from build123d import *

# Parameters (mm, degrees)
PAD_DEPTH         = 50
SKETCH001_W       = 0.9
SKETCH001_H       = 10
POCKET_DEPTH      = 10.001
POCKET_DEPTH_BACK = -10.001
CHAMFER_SIZE      = 1
CHAMFER001_SIZE   = 0.5


with BuildPart() as part:
    # Sketch → Pad (new body)
    with BuildSketch(Plane.YZ):
        with BuildLine():
            Line((-10, 0), (10, 0))
            Line((10, 0), (7.5, 10))
            Line((7.5, 10), (2.3, 10))
            Line((2.3, 10), (1.906144, 6.463458))
            ThreePointArc((1.906144, 6.463458), (1.913219, 6.190714), (1.99375, 5.930033))
            ThreePointArc((-1.99375, 5.930033), (0, 2.8), (1.99375, 5.930033))
            ThreePointArc((-1.99375, 5.930033), (-1.913219, 6.190714), (-1.906144, 6.463458))
            Line((-1.906144, 6.463458), (-2.3, 10))
            Line((-2.3, 10), (-7.5, 10))
            Line((-7.5, 10), (-10, 0))
        make_face()
    extrude(amount=PAD_DEPTH)

    # Sketch001 → Pocket (cut, two sides)
    with BuildSketch(Plane.XZ) as pocket_sk:
        with Locations((10.45, 7)):
            Rectangle(SKETCH001_W, SKETCH001_H)
    extrude(amount=-POCKET_DEPTH, mode=Mode.SUBTRACT)
    extrude(pocket_sk.sketch, amount=-POCKET_DEPTH_BACK, mode=Mode.SUBTRACT)

    # Chamfer
    chamfer_edges = [part.edges().sort_by_distance(p)[0] for p in [
        (25, 10, 0),
        (25, -10, 0),
    ]]
    chamfer(chamfer_edges, length=CHAMFER_SIZE)

    # Chamfer001
    chamfer001_edges = [part.edges().sort_by_distance(p)[0] for p in [
        (50, -8.628732, 5.485071),
        (50, -9.378732, 0.485071),
        (50, -4.9, 10),
        (50, 0, 0),
        (50, -2.103072, 8.231729),
        (50, 9.378732, 0.485071),
        (50, -1.913219, 6.190714),
        (50, 8.628732, 5.485071),
        (50, 0, 2.8),
        (50, 4.9, 10),
        (50, 1.913219, 6.190714),
        (50, 2.103072, 8.231729),
        (0, -8.628732, 5.485071),
        (0, -9.378732, 0.485071),
        (0, -4.9, 10),
        (0, 0, 0),
        (0, -2.103072, 8.231729),
        (0, 9.378732, 0.485071),
        (0, -1.913219, 6.190714),
        (0, 8.628732, 5.485071),
        (0, 0, 2.8),
        (0, 4.9, 10),
        (0, 1.913219, 6.190714),
        (0, 2.103072, 8.231729),
        (5, -7.5, 10),
        (10, -4.9, 10),
        (5, -2.3, 10),
        (5, 2.3, 10),
        (10, 4.9, 10),
        (5, 7.5, 10),
        (10.9, 4.9, 10),
        (30.45, 2.3, 10),
        (30.45, 7.5, 10),
        (10.9, -4.9, 10),
        (30.45, -7.5, 10),
        (30.45, -2.3, 10),
        (10, -8.5, 6),
        (10, 8.5, 6),
        (10.9, 8.5, 6),
        (10.9, -8.5, 6),
    ]]
    chamfer(chamfer001_edges, length=CHAMFER001_SIZE)


solid = part.part
Model file for the job. Use its own axes, mm. A direction names the side the tool comes from. Give positions to 0.01 mm unless a question says otherwise; leave off trailing zeros. Loops run counter-clockwise (first coordinate to the right, second up) from the corner with the lowest first, then second, coordinate; pieces in that order, holes last.
1) Pull direction X, two halves, no side cores. Call faces 4 (the flat face through (30, -5, 10)), 5 (the flat face through (11.146, 8.315, 5.696)), 6 (the flat face through (49.754, 9.174, 0.634)): +X half, -X half, draft (parallel to the pull), parting line (faces both ways), or undercut.
2) Wall check: line 1 (X direction, y = 4.25, z = 8.25); line 2 (Y direction, x = 8, z = 5); line 3 (Z direction, x = 38, y = 0). Give the ranges that are in metal, low to high.
3) Saw through at C-C (y = -3.25). Write the cut outline in (x, z), plus the area to 3 significant figures.
4) Saw through at A-A (z = 5). Write the cut outline in (x, y), plus the area to 3 significant figures.
5) Tool access for faces 1 (the flat face through (0, 0, 2)), 2 (the flat face through (5.184, -2.073, 7.962)), 3 (the flat face through (10, 2.1, 6.5)): list every direction of +Z, -Z, +X, -X, +Y, -Y with a clear straight run to the whole face (end or side of a thin tool).
6) Saw through at B-B (x = 13.5). Write the cut outline in (y, z).
7) Saw through at D-D (z = 8.25). Write the cut outline in (x, y).
8) Flat gauge pins, fed straight in: pin 1 Ø6 at (x, z) = (40, 8.5) entering from +Y (3 decimals); pin 2 Ø1 at (x, z) = (6.5, 8.5) entering from +Y; pin 3 Ø4 at (x, y) = (34, -1.5) entering from +Z; pin 4 Ø2 at (x, z) = (16, 7) entering from +Y. Where does each tip first touch, or does it go through?
Answer block:
1. face 4: draft
1. face 5: undercut
1. face 6: +X half
2. line 1: x = 0 to 10, 10.9 to 50
2. line 2: y = -8.75 to -2.2, 2.2 to 8.75
2. line 3: z = 0 to 2.8
3. outline: (0, 0.5) - (0.5, 0) - (49.5, 0) - (50, 0.5) - (50, 9.5) - (49.5, 10) - (11.4, 10) - (10.9, 9.5) - (10.9, 2) - (10, 2) - (10, 9.5) - (9.5, 10) - (0.5, 10) - (0, 9.5) - close
3. area: 492 mm2
4. outline: (0, -8.23) - (0.5, -8.75) - (9.5, -8.75) - (10, -8.23) - (10, -2.2) - (0.5, -2.2) - (0, -2.7) - close; (0, 2.7) - (0.5, 2.2) - (10, 2.2) - (10, 8.23) - (9.5, 8.75) - (0.5, 8.75) - (0, 8.23) - close; (10.9, -8.23) - (11.4, -8.75) - (49.5, -8.75) - (50, -8.23) - (50, -2.7) - (49.5, -2.2) - (10.9, -2.2) - close; (10.9, 2.2) - (49.5, 2.2) - (50, 2.7) - (50, 8.23) - (49.5, 8.75) - (11.4, 8.75) - (10.9, 8.23) - close
4. area: 642 mm2
5. face 1: +Z, -Z, -X, +Y, -Y
5. face 2: +Z, +X, -X
5. face 3: +Z, +Y, -Y
6. outline: (-9.76, 0.97) - (-9, 0) - (9, 0) - (9.76, 0.97) - (7.62, 9.51) - (7, 10) - (2.8, 10) - (2.24, 9.5) - (1.91, 6.46) arc R1 ccw to (1.99, 5.93) arc R2.2 cw (long way) to (-1.99, 5.93) arc R1 ccw to (-1.91, 6.46) - (-2.24, 9.5) - (-2.8, 10) - (-7, 10) - (-7.62, 9.51) - close
7. outline: (0, -7.42) - (0.5, -7.94) - (9.5, -7.94) - (10, -7.42) - (10, -2.11) - (0.5, -2.11) - (0, -2.61) - close; (0, 2.61) - (0.5, 2.11) - (10, 2.11) - (10, 7.42) - (9.5, 7.94) - (0.5, 7.94) - (0, 7.42) - close; (10.9, -7.42) - (11.4, -7.94) - (49.5, -7.94) - (50, -7.42) - (50, -2.61) - (49.5, -2.11) - (10.9, -2.11) - close; (10.9, 2.11) - (49.5, 2.11) - (50, 2.61) - (50, 7.42) - (49.5, 7.94) - (11.4, 7.94) - (10.9, 7.42) - close
8. pin 1: stops at y = 8.625
8. pin 2: stops at y = 8
8. pin 3: stops at z = 10
8. pin 4: stops at y = 8.5
